Geometry check sheet. Reference: drawing and pictorial views, mm from the part's lowest x, y, z. A direction names the side the tool comes from. Round coordinates to 2 decimals unless told otherwise and drop trailing zeros. Write each loop counter-clockwise with the first axis right and the second up, starting at its lowest first coordinate (ties: lowest second). Pieces come first, ordered by that corner, then holes. Notation, with made-up numbers: (16, 73) -> (41, 73) arc R26 cw to (41, 90) -> close; hole circle Ø1 at (70, 77.25). An arc over 180 degrees is marked (long way). Answer as a JSON object with one key per item and string values. Group by question number.
(1) Gauge pin test, flat ends, axial feed: pin 1 Ø2.5 at (x, y) = (17.95, 7.2) entering from -Z; pin 2 Ø5 at (x, y) = (7, 6) entering from -Z; pin 3 Ø2.5 at (x, y) = (16.5, 6.5) entering from -Z. Record the tip position at first contact, or that the pin passes through.
(2) Set-up check for the marked faces 4 and 5: record each of +Z, -Z, +X, -X, +Y, -Y from which the full face is reachable in a straight line by a thin tool's end or side.
(3) Sectioned sample at C-C on x = 12. Record the cut outline in (y, z).
(4) Scan lines: L1, parallel to Y at x = 17.95, z = 1.3; L2, parallel to Y at x = 12, z = 0.9; L3, parallel to X at y = 8, z = 0.85 (1 decimal). Record each from-to range of solid material in increasing order. Write a range as from..to.
(5) Sectioned sample at A-A on y = 7.2. Record the cut outline in (x, z).
(6) Sectioned sample at D-D on y = 4.5. Record the cut outline in (x, z).
(7) Sectioned sample at B-B on z = 0.55. Record the cut outline in (x, y), and give its area (3 significant figures).
(8) Draft check along Y on the marked faces 1, 2 and 3. Enter one of: released by +Y, released by -Y, zero draft, split by the parting line, or undercut.
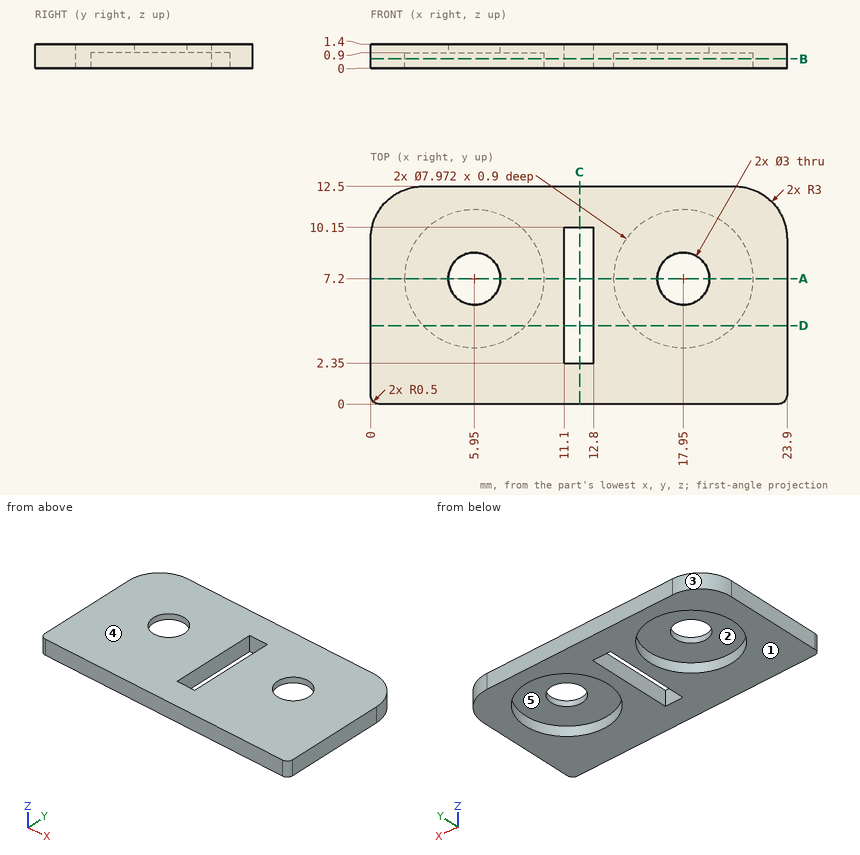
Computed values:
{
 "1": {"pin 1": "through", "pin 2": "z = 0", "pin 3": "z = 0.9"},
 "2": {"face 4": "+Z, +X, -X, +Y, -Y", "face 5": "-Z"},
 "3": {"outline": "(0, 0) -> (2.35, 0) -> (2.35, 1.4) -> (0, 1.4) -> close; (10.15, 0) -> (12.5, 0) -> (12.5, 1.4) -> (10.15, 1.4) -> close"},
 "4": {"L1": "0..5.7, 8.7..12.5", "L2": "0..2.35, 10.15..12.5", "L3": "0..2, 9.9..11.1, 12.8..14, 21.9..23.9"},
 "5": {"outline": "(0, 0) -> (1.96, 0) -> (1.96, 0.9) -> (4.45, 0.9) -> (4.45, 1.4) -> (0, 1.4) -> close; (7.45, 0.9) -> (9.94, 0.9) -> (9.94, 0) -> (11.1, 0) -> (11.1, 1.4) -> (7.45, 1.4) -> close; (12.8, 0) -> (13.96, 0) -> (13.96, 0.9) -> (16.45, 0.9) -> (16.45, 1.4) -> (12.8, 1.4) -> close; (19.45, 0.9) -> (21.94, 0.9) -> (21.94, 0) -> (23.9, 0) -> (23.9, 1.4) -> (19.45, 1.4) -> close"},
 "6": {"outline": "(0, 0) -> (3.02, 0) -> (3.02, 0.9) -> (8.88, 0.9) -> (8.88, 0) -> (11.1, 0) -> (11.1, 1.4) -> (0, 1.4) -> close; (12.8, 0) -> (15.02, 0) -> (15.02, 0.9) -> (20.88, 0.9) -> (20.88, 0) -> (23.9, 0) -> (23.9, 1.4) -> (12.8, 1.4) -> close"},
 "7": {"outline": "(0, 0.5) arc R0.5 ccw to (0.5, 0) -> (23.4, 0) arc R0.5 ccw to (23.9, 0.5) -> (23.9, 9.5) arc R3 ccw to (20.9, 12.5) -> (3, 12.5) arc R3 ccw to (0, 9.5) -> close; hole circle Ø7.97 at (5.95, 7.2); hole (11.1, 2.35) -> (12.8, 2.35) -> (12.8, 10.15) -> (11.1, 10.15) -> close; hole circle Ø7.97 at (17.95, 7.2)", "area": "182 mm2"},
 "8": {"face 1": "zero draft", "face 2": "undercut", "face 3": "released by +Y"}
}
